Design review of the part built by this model. Coordinates are the model's own, in mm. A direction names the side the tool comes from. Coordinates: 2 decimals unless noted, no trailing zeros. Write each loop counter-clockwise with the first axis right and the second up, starting at its lowest first coordinate (ties: lowest second). Pieces come first, ordered by that corner, then holes. Notation, with made-up numbers: M 42,17.25 L 55,17.25 A16 cw 55,28.25 Z; hole C 44,-15 d6. An arc over 180 degrees is marked long. Write item = value, one per line.
```python
from build123d import *

# Parameters (mm, degrees)
SKETCH1_W                = 30
SKETCH1_H                = 30
BASE_PLATE_DEPTH         = 1.5
SIDE_WALLS_DEPTH         = 6
SKETCH3_W                = 10
SKETCH3_H                = 30
SWITCH_BLOCK_DEPTH       = 9.5
SKETCH11_W               = 8.5
SKETCH11_H               = 30
SKETCH11_W_2             = 11.5
THICKER_BODY_DEPTH       = 2.5
SWITCH_BLOCK_ANGLE_DEPTH = 30
SKETCH6_W                = 6.25
SKETCH6_H                = 13.25
SWITCH_POCKET_DEPTH      = 6.75
WIRE_CHANNEL_1_REACH     = 33.348
SKETCH7_W                = 2.75
SKETCH7_H                = 13.25
SKETCH19_W               = 2.79179182
SKETCH19_H               = 13.25
SWITCH_REMOVER_DEPTH     = 10
SKETCH4_R                = 1.625
M2_SCREWS_DEPTH          = 6
M2_NUTS_DEPTH            = 2
SKETCH17_R               = 1.65
M3_MOUNTING_SCREWS_DEPTH = 31.960660523
WIRE_CHANNEL_REACH       = 32.267
SKETCH8_W                = 8
SKETCH8_H                = 3.25
FILLET1_R                = 1
FILLET2_R                = 0.5
FILLET3_R                = 0.5
FILLET4_R                = 0.75
FILLET5_R                = 0.75


with BuildPart() as part:
    # Sketch1 → Base Plate (new body)
    with BuildSketch(Plane(origin=(0, 0, 0), x_dir=(1, 0, 0), z_dir=(0, 1, 0))):
        Rectangle(SKETCH1_W, SKETCH1_H)
    extrude(amount=BASE_PLATE_DEPTH)

    # Sketch2 → Side Walls (add)
    with BuildSketch(Plane.XZ):
        Polygon((15, 15), (-15, 15), (-15, -15), (15, -15), (15, -21), (-21, -21), (-21, 21), (15, 21), align=None)
    extrude(amount=-SIDE_WALLS_DEPTH)

    # Sketch3 → Switch Block (add)
    with BuildSketch(Plane(origin=(0, 1.5, 0), x_dir=(1, 0, 0), z_dir=(0, 1, 0))):
        with Locations((-1.5, 0)):
            Rectangle(SKETCH3_W, SKETCH3_H)
    extrude(amount=SWITCH_BLOCK_DEPTH)

    # Sketch11 → Thicker Body (add)
    with BuildSketch(Plane(origin=(0, 1.5, 0), x_dir=(1, 0, 0), z_dir=(0, 1, 0))):
        with Locations((-10.75, 0)):
            Rectangle(SKETCH11_W, SKETCH11_H)
        with Locations((9.25, 0)):
            Rectangle(SKETCH11_W_2, SKETCH11_H)
    extrude(amount=THICKER_BODY_DEPTH)

    # Sketch5 → Switch Block Angle (add)
    with BuildSketch(Plane(origin=(0, 0, -15), x_dir=(-1, 0, 0), z_dir=(0, 0, -1))):
        Polygon((6.5, 11), (6.5, 12.75), (-3.5, 11), align=None)
    extrude(amount=-SWITCH_BLOCK_ANGLE_DEPTH)

    # Sketch6 → Switch Pocket (cut)
    with BuildSketch(Plane(origin=(1.971801092, 11.267434809, 0), x_dir=(0.9850304671557043, -0.17238033175224804, 0), z_dir=(0.17238033175224804, 0.9850304671557043, 0))):
        with Locations((-3.52456214, 0)):
            Rectangle(SKETCH6_W, SKETCH6_H)
    extrude(amount=-SWITCH_POCKET_DEPTH, mode=Mode.SUBTRACT)

    # Wire Channel 1: up to this plane
    wire_channel_1_end = Plane(origin=(0, 1, 0), z_dir=(0, 1, 0))
    # Sketch7 → Wire Channel 1 (cut, up to the surface)
    with BuildSketch(Plane(origin=(0.808233852, 4.618479156, 0), x_dir=(0.9850304671557043, -0.17238033175224815, 0), z_dir=(0.17238033175224815, 0.9850304671557043, 0)), mode=Mode.PRIVATE) as wire_channel_1_sk1:
        with Locations((-3.52456214, 0)):
            Rectangle(SKETCH7_W, SKETCH7_H)
    wire_channel_1_tool1 = split(extrude(wire_channel_1_sk1.sketch, amount=-WIRE_CHANNEL_1_REACH, mode=Mode.PRIVATE), bisect_by=wire_channel_1_end, keep=Keep.BOTH, mode=Mode.PRIVATE)
    add(wire_channel_1_tool1.solids().sort_by_distance((-2.663567, 5.226044, 0))[0], mode=Mode.SUBTRACT)

    # Sketch19 → Switch Remover (cut)
    with BuildSketch(Plane(origin=(0, 1, 0), x_dir=(1, 0, 0), z_dir=(0, 1, 0))):
        with Locations((-3.403125, 0)):
            Rectangle(SKETCH19_W, SKETCH19_H)
    extrude(amount=-SWITCH_REMOVER_DEPTH, mode=Mode.SUBTRACT)

    # Sketch4 → M2 Screws (cut)
    with BuildSketch(Plane(origin=(0, 6, 0), x_dir=(1, 0, 0), z_dir=(0, 1, 0))):
        with Locations(Location((-16, -18, 0), (0, 0, 270))):
            Circle(SKETCH4_R)
        with Locations(Location((10, -18, 0), (0, 0, 270))):
            Circle(SKETCH4_R)
        with Locations(Location((10, 18, 0), (0, 0, 270))):
            Circle(SKETCH4_R)
        with Locations(Location((-16, 18, 0), (0, 0, 270))):
            Circle(SKETCH4_R)
    extrude(amount=-M2_SCREWS_DEPTH, mode=Mode.SUBTRACT)

    # Sketch16 → M2 Nuts (cut)
    with BuildSketch(Plane.XZ):
        Polygon((-14.773130678, 15.875), (-13.546261356, 18), (-14.773130678, 20.125), (-17.226869322, 20.125), (-18.453738644, 18), (-17.226869322, 15.875), align=None)
        Polygon((-17.226869322, -15.875), (-14.773130678, -15.875), (-13.546261356, -18), (-14.773130678, -20.125), (-17.226869322, -20.125), (-18.453738644, -18), align=None)
        Polygon((11.226869322, 15.875), (12.453738644, 18), (11.226869322, 20.125), (8.773130678, 20.125), (7.546261356, 18), (8.773130678, 15.875), align=None)
        Polygon((8.773130678, -15.875), (11.226869322, -15.875), (12.453738644, -18), (11.226869322, -20.125), (8.773130678, -20.125), (7.546261356, -18), align=None)
    extrude(amount=-M2_NUTS_DEPTH, mode=Mode.SUBTRACT)

    # Sketch17 → M3 Mounting Screws (cut, through all)
    with BuildSketch(Plane(origin=(0, 4, 0), x_dir=(1, 0, 0), z_dir=(0, 1, 0))):
        with Locations(Location((7.078853568, 10, 0), (0, 0, 270))):
            Circle(SKETCH17_R)
        with Locations(Location((7.078853568, -10, 0), (0, 0, 270))):
            Circle(SKETCH17_R)
        with Locations(Location((-10.75, -10, 0), (0, 0, 270))):
            Circle(SKETCH17_R)
        with Locations(Location((-10.75, 10, 0), (0, 0, 270))):
            Circle(SKETCH17_R)
    extrude(amount=-M3_MOUNTING_SCREWS_DEPTH, mode=Mode.SUBTRACT)

    # M3 Heads cone 1 section (through the dimple's axis) → M3 Heads (revolve, cut)
    with BuildSketch(Plane(origin=(7.078853568, 4, -10), x_dir=(0, 0, 1), z_dir=(1, 0, 0))):
        Polygon((0, 0), (3.25, 0), (0, 3.25), align=None)
    revolve(axis=Axis((7.078853568, 4, -10), (0, -1, 0)), mode=Mode.SUBTRACT)

    # M3 Heads cone 2 section (through the dimple's axis) → M3 Heads cone 2 (revolve, cut)
    with BuildSketch(Plane(origin=(7.078853568, 4, 10), x_dir=(0, 0, 1), z_dir=(1, 0, 0))):
        Polygon((0, 0), (3.25, 0), (0, 3.25), align=None)
    revolve(axis=Axis((7.078853568, 4, 10), (0, -1, 0)), mode=Mode.SUBTRACT)

    # M3 Heads cone 3 section (through the dimple's axis) → M3 Heads cone 3 (revolve, cut)
    with BuildSketch(Plane(origin=(-10.75, 4, 10), x_dir=(0, 0, 1), z_dir=(1, 0, 0))):
        Polygon((0, 0), (3.25, 0), (0, 3.25), align=None)
    revolve(axis=Axis((-10.75, 4, 10), (0, -1, 0)), mode=Mode.SUBTRACT)

    # M3 Heads cone 4 section (through the dimple's axis) → M3 Heads cone 4 (revolve, cut)
    with BuildSketch(Plane(origin=(-10.75, 4, -10), x_dir=(0, 0, 1), z_dir=(1, 0, 0))):
        Polygon((0, 0), (3.25, 0), (0, 3.25), align=None)
    revolve(axis=Axis((-10.75, 4, -10), (0, -1, 0)), mode=Mode.SUBTRACT)

    # Wire Channel: up to this face of the body (flat: up to its plane)
    wire_channel_end = Plane(part.part.faces().sort_by_distance((-21, 3, 0))[0])
    # Sketch8 → Wire Channel (cut, up to the picked face)
    with BuildSketch(Plane(origin=(-4.017984132, 2.099725317, 0), x_dir=(0, 0, 1), z_dir=(-1, 0, 0)), mode=Mode.PRIVATE) as wire_channel_sk1:
        with Locations((0, 0.275274683)):
            Rectangle(SKETCH8_W, SKETCH8_H)
    wire_channel_tool1 = split(extrude(wire_channel_sk1.sketch, amount=WIRE_CHANNEL_REACH, mode=Mode.PRIVATE), bisect_by=wire_channel_end, keep=Keep.BOTH, mode=Mode.PRIVATE)
    add(wire_channel_tool1.solids().sort_by(Axis((-4.017984, 2.375, 0), (-1, 0, 0)))[0], mode=Mode.SUBTRACT)

    # Fillet1
    fillet1_edges = [part.edges().sort_by_distance(p)[0] for p in [
        (-6.5, 12.75, 0),
    ]]
    fillet(fillet1_edges, radius=FILLET1_R)

    # Fillet2
    fillet2_edges = [part.edges().sort_by_distance(p)[0] for p in [
        (15, 3, 21),
    ]]
    fillet(fillet2_edges, radius=FILLET2_R)

    # Fillet3
    fillet3_edges = [part.edges().sort_by_distance(p)[0] for p in [
        (15, 3, -21),
    ]]
    fillet(fillet3_edges, radius=FILLET3_R)

    # Fillet4
    fillet4_edges = [part.edges().sort_by_distance(p)[0] for p in [
        (-21, 3, -21),
    ]]
    fillet(fillet4_edges, radius=FILLET4_R)

    # Fillet5
    fillet5_edges = [part.edges().sort_by_distance(p)[0] for p in [
        (-21, 3, 21),
    ]]
    fillet(fillet5_edges, radius=FILLET5_R)


solid = part.part
```
Q1. For P1, Ø8, axis at x = -5, z = -3.5, coming from the +Y side; P2, Ø11, axis at x = 0.5, z = -10, coming from the +Y side; P3, Ø1.5, axis at x = -5, y = 10, coming from the -Z side; P4, Ø1.5, axis at y = 9.5, z = -6, coming from the +X side, all flat-tipped, find the tip position at first contact; note any pin that passes through.
Check result:
P1 = 12.56
P2 = 12.49
P3 = -15
P4 = 3.5
Q2. The part is to be moulded in two halves that separate along X. For faces 1 (the flat face through (-5, 4, 0)), 2 (the flat face through (-4.892, 5.616, -0.093)), say which applies: +X half, -X half, draft (parallel to the pull), parting line (faces both ways), or undercut.
Check result:
face_1 = draft
face_2 = undercut
Q3. Consider section B-B, the plane z = -2. State the section outline as (x, y) points.
Check result:
outline = M -21,0 L -4.8,0 L -4.8,0.75 L -21,0.75 Z; M -21,4 L -15,4 L -15,6 L -21,6 Z; M -6.5,4 L -4.27,4 L -4.02,5.46 L -5.74,5.76 L -4.58,12.41 L -5.33,12.54 A1 ccw -6.5,11.56 Z; M -2.01,0 L 15,0 L 15,4 L 3.5,4 L 3.5,11 L 1.58,11.34 L 0.41,4.69 L -1.31,4.99 L -2.01,1 Z
Q4. Machinability: for faces 3 (the flat face through (-1, 9, -15)), 4 (the flat face through (-1.653, 3.022, 0.093)), 5 (the flat face through (11.83, 0.99, 16.92)), which of the approach directions +Z, -Z, +X, -X, +Y, -Y give a long, thin tool a straight path to every point of the face, cutting with its end or side? Answer none if there is none.
Check result:
face_3 = -Z, +X, -X, +Y
face_4 = +Y
face_5 = -Y
Q5. Consider section A-A, the plane x = -16. State the section outline as (y, z) points (3 decimals).
Check result:
outline = M 0,-21 L 6,-21 L 6,-19.625 L 2,-19.625 L 2,-20.125 L 0,-20.125 Z; M 0,-15.875 L 2,-15.875 L 2,-16.375 L 6,-16.375 L 6,16.375 L 2,16.375 L 2,15.875 L 0,15.875 Z; M 0,20.125 L 2,20.125 L 2,19.625 L 6,19.625 L 6,21 L 0,21 Z; hole M 0.75,-4 L 4,-4 L 4,4 L 0.75,4 Z
Q6. Consider section C-C, the plane z = -10. State the section outline as (x, y) points, and give its area (3 significant figures).
Check result:
outline = M -21,0 L -12.4,0 L -12.4,2.4 L -14,4 L -15,4 L -15,6 L -21,6 Z; M -9.1,0 L 5.43,0 L 5.43,2.4 L 3.83,4 L 3.5,4 L 3.5,11 L -5.33,12.54 A1 ccw -6.5,11.56 L -6.5,4 L -7.5,4 L -9.1,2.4 Z; M 8.73,0 L 15,0 L 15,4 L 10.33,4 L 8.73,2.4 Z
area = 203 mm²
Q7. Consider section D-D, the plane y = 6.75. State the section outline as (x, z) points (3 decimals).
Check result:
outline = M -6.5,-15 L 3.5,-15 L 3.5,15 L -6.5,15 Z; hole M -5.569,-6.625 L 0.776,-6.625 L 0.776,6.625 L -5.569,6.625 Z
Q8. Wall thickness on line 1 (X direction, y = 0.6, z = -10); line 2 (Z direction, x = 9.5, y = 1.5) (3 decimals); line 3 (X direction, y = 4.5, z = 18) (3 decimals): over which ranges is each line inside the solid? List them lowest first.
Check result:
line_1 = -21 to -12.4, -9.1 to 5.43, 8.73 to 15
line_2 = -21 to -20.125, -15.875 to 15.875, 20.125 to 21
line_3 = -21 to -17.625, -14.375 to 8.375, 11.625 to 15
